```python
from build123d import *

# Parameters (mm, degrees)
SKETCH1_R           = 48
SKETCH1_R_2         = 44
BOSS_EXTRUDE1_DEPTH = 6
CUT_EXTRUDE3_START  = 1
SKETCH2_R           = 47.15
SKETCH2_R_2         = 45.05
CUT_EXTRUDE3_DEPTH  = 10
SKETCH3_R           = 1.5
BOSS_EXTRUDE2_DEPTH = 7
FILLET1_R           = 0.1


with BuildPart() as part:
    # Sketch1 → Boss-Extrude1 (new body)
    with BuildSketch(Plane(origin=(0, 0, 0), x_dir=(1, 0, 0), z_dir=(0, 1, 0))):
        Circle(SKETCH1_R)
        Circle(SKETCH1_R_2, mode=Mode.SUBTRACT)
    extrude(amount=BOSS_EXTRUDE1_DEPTH)

    # Sketch2 → Cut-Extrude3 (cut)
    with BuildSketch(Plane(origin=(0, 0, 0), x_dir=(1, 0, 0), z_dir=(0, 1, 0)).offset(CUT_EXTRUDE3_START)):
        Circle(SKETCH2_R)
        Circle(SKETCH2_R_2, mode=Mode.SUBTRACT)
    extrude(amount=CUT_EXTRUDE3_DEPTH, mode=Mode.SUBTRACT)

    # Sketch3 → Boss-Extrude2 (add)
    with BuildSketch(Plane(origin=(0, 0, 0), x_dir=(1, 0, 0), z_dir=(0, 1, 0))):
        with Locations((0, 47)):
            Circle(SKETCH3_R)
        with Locations((47, 0)):
            Circle(SKETCH3_R)
        with Locations((-0.045212766, -46.999978253)):
            Circle(SKETCH3_R)
        with Locations((-46.999978253, -0.045212766)):
            Circle(SKETCH3_R)
    extrude(amount=-BOSS_EXTRUDE2_DEPTH)

    # Fillet1
    fillet1_edges = [part.edges().sort_by_distance(p)[0] for p in [
        (-1.5, -7, -47),
        (45.5, -7, 0),
        (-1.545212766, -7, 46.999978253),
        (-48.499978253, -7, 0.045212766),
    ]]
    fillet(fillet1_edges, radius=FILLET1_R)


solid = part.part
```
Geometry check sheet. Reference: the model listing, model coordinates, mm. A direction names the side the tool comes from. Round coordinates to 2 decimals unless told otherwise and drop trailing zeros. Loops run counter-clockwise (first coordinate to the right, second up) from the corner with the lowest first, then second, coordinate; pieces in that order, holes last. Notation, with made-up numbers: (59, 29.25) - (70, 29.25) arc R23 cw to (70, 46.25) - close; hole circle Ø10 at (52, -1.5). An arc over 180 degrees is marked (long way). Use a Markdown table: item, result.
Q1. Cross-section at B-B on x = 35. Record the cut outline in (y, z), plus the area to 3 significant figures.
Solutions:
| item | result |
|---|---|
| outline | (0, -32.85) - (6, -32.85) - (6, -31.59) - (1, -31.59) - (1, -28.36) - (6, -28.36) - (6, -26.66) - (0, -26.66) - close; (0, 26.66) - (6, 26.66) - (6, 28.36) - (1, 28.36) - (1, 31.59) - (6, 31.59) - (6, 32.85) - (0, 32.85) - close |
| area | 41.9 mm2 |
Q2. Cross-section at C-C on y = 2.25. Record the cut outline in (x, z).
Solutions:
| item | result |
|---|---|
| outline | circle Ø96 at (0, 0); circle Ø90.1 at (0, 0); hole circle Ø94.3 at (0, 0); hole circle Ø88 at (0, 0) |
Q3. Material ranges on line 1 (X direction, y = 3.65, z = 0); line 2 (X direction, y = 1.25, z = 20), recorded low to high.
Solutions:
| item | result |
|---|---|
| line 1 | x = -48 to -47.15, -45.05 to -44, 44 to 45.05, 47.15 to 48 |
| line 2 | x = -43.63 to -42.7, -40.37 to -39.19, 39.19 to 40.37, 42.7 to 43.63 |
Q4. Go/stop test with flat-tipped pins: P1, Ø4, axis at x = -10, y = -1, coming from the +Z side; P2, Ø1.5, axis at x = 35, z = 26.5, coming from the +Y side; P3, Ø2, axis at y = 3, z = 8, coming from the -X side; P4, Ø2, axis at x = 33.5, y = 4, coming from the -Z side. Record where each tip stops, or that it passes through.
Solutions:
| item | result |
|---|---|
| P1 | stops at z = 47.28 |
| P2 | stops at y = 6 |
| P3 | stops at x = -47.49 |
| P4 | stops at z = -35.32 |
Q5. Cross-section at D-D on y = -4. Record the cut outline in (x, z).
Solutions:
| item | result |
|---|---|
| outline | circle Ø3 at (-47, 0.05); circle Ø3 at (-0.05, 47); circle Ø3 at (0, -47); circle Ø3 at (47, 0) |
Q6. Access from +Z, -Z, +X, -X, +Y, -Y to the whole of each face (thin tool, end or side, straight path). Record for faces 1 (the flat face through (0, -7, 47)), 2 (the flat face through (38.2, 1, 24.2)), 3 (the cylindrical face through (45.5, -3.4, -0.07)).
Solutions:
| item | result |
|---|---|
| face 1 | +Z, -Z, +X, -X, -Y |
| face 2 | +Y |
| face 3 | -Y |
Q7. Draft check along Z on faces 4 (the flat face through (9.8, 6, 43.2)), 5 (the cylindrical face through (-45.57, -3.4, -0.41)), 6 (the cylindrical face through (-9.538, 2.958, 42.954)). Enter one of: released by +Z, released by -Z, zero draft, split by the parting line, or undercut.
Solutions:
| item | result |
|---|---|
| face 4 | zero draft |
| face 5 | split by the parting line |
| face 6 | undercut |
Q8. Cross-section at A-A on z = -3. Record the cut outline in (x, y), plus the area to 3 significant figures.
Solutions:
| item | result |
|---|---|
| outline | (-47.91, 0) - (-43.9, 0) - (-43.9, 6) - (-44.95, 6) - (-44.95, 1) - (-47.05, 1) - (-47.05, 6) - (-47.91, 6) - close; (43.9, 0) - (47.91, 0) - (47.91, 6) - (47.05, 6) - (47.05, 1) - (44.95, 1) - (44.95, 6) - (43.9, 6) - close |
| area | 27.1 mm2 |
